Input: part model. Units: mm. Frame: model coordinates. A direction names the side the tool comes from. Give positions to 0.01 mm unless a question says otherwise; leave off trailing zeros. Order: outer loops, then holes, each group sorted by start corner. A loop starts at its lowest first (then second) coordinate and runs counter-clockwise, first axis right, second up. Notation, with made-up numbers: M -10.5,24 L 4.5,24 A31 cw 4.5,60 Z; hole C 60.5,29.5 d2. An arc over 180 degrees is marked long. Use a Markdown table: item, result.
from build123d import *

# Parameters (mm, degrees)
F0_W     = 45
F0_H     = 131
F1_DEPTH = 2
F2_W     = 45
F2_H     = 131
F3_DEPTH = 5
F5_W     = 35
F5_H     = 100
F6_DEPTH = 4
F7_W     = 5
F7_H     = 100
F8_DEPTH = 2
F4_W     = 15
F4_H     = 90
F9_DEPTH = 7.001


with BuildPart() as f1:
    # F0 (on Top) → F1 (new body)
    with BuildSketch(Plane.XY):
        with Locations((22.5, 65.5)):
            Rectangle(F0_W, F0_H)
    extrude(amount=F1_DEPTH)

    # F2 (on face) → F3 (join)
    with BuildSketch(Plane.XY.offset(2)):
        with Locations((22.5, 65.5)):
            Rectangle(F2_W, F2_H)
    extrude(amount=F3_DEPTH)

    # F5 (on face) → F6 (cut)
    with BuildSketch(Plane.XY.offset(7)):
        with Locations((22.5, 71)):
            Rectangle(F5_W, F5_H)
    extrude(amount=-F6_DEPTH, mode=Mode.SUBTRACT)

    # F7 (on face) → F8 (join)
    with BuildSketch(Plane.XY.offset(3)):
        with Locations((22.5, 71)):
            Rectangle(F7_W, F7_H)
    extrude(amount=F8_DEPTH)

    # F4 (on face) → F9 (cut, through all)
    with BuildSketch(Plane.XY.offset(7)):
        with Locations((22.5, 71)):
            Rectangle(F4_W, F4_H)
    extrude(amount=-F9_DEPTH, mode=Mode.SUBTRACT)


solid = f1.part
1) First-contact query: pin 1 Ø12 at (x, y) = (33, 68.5) entering from +Z; pin 2 Ø4 at (x, y) = (23.5, 118) entering from +Z. Flat tips, straight axial feed; report the tip coordinate or a pass-through.
Response values:
| item | result |
|---|---|
| pin 1 | stops at z = 3 |
| pin 2 | stops at z = 5 |
2) Material intervals for line 1 (X direction, y = 118.5, z = 4); line 2 (X direction, y = 102.5, z = 1.75); line 3 (Y direction, x = 22.5, z = 6.5), sorted ascending. Write a range as from..to.
Response values:
| item | result |
|---|---|
| line 1 | x = 0..5, 20..25, 40..45 |
| line 2 | x = 0..15, 30..45 |
| line 3 | y = 0..21, 121..131 |
3) Cut plane A-A on x = 28.5. Return loops of the section in (y, z), and give its area (3 significant figures).
Response values:
| item | result |
|---|---|
| outline | M 0,0 L 26,0 L 26,3 L 21,3 L 21,7 L 0,7 Z; M 116,0 L 131,0 L 131,7 L 121,7 L 121,3 L 116,3 Z |
| area | 247 mm² |
4) Cut plane B-B on y = 93. Return loops of the section in (x, z).
Response values:
| item | result |
|---|---|
| outline | M 0,0 L 15,0 L 15,3 L 5,3 L 5,7 L 0,7 Z; M 30,0 L 45,0 L 45,7 L 40,7 L 40,3 L 30,3 Z |
5) Mould query, pull axis Y, two halves, no side actions, for faces 4 (the face through (22, 0, 3)), 5 (the face through (11, 72, 3)), 6 (the face through (22, 131, 3)). Classes: released by +Y, released by -Y, zero draft, split by the parting line, or undercut.
Response values:
| item | result |
|---|---|
| face 4 | released by -Y |
| face 5 | undercut |
| face 6 | released by +Y |
6) Reachability of faces 1 (the face through (12, 66, 0)), 2 (the face through (22, 116, 2)), 3 (the face through (22.3, 121, 5.5)) from +Z, -Z, +X, -X, +Y, -Y: full face, straight path, thin tool, end or side. Return the list, or none.
Response values:
| item | result |
|---|---|
| face 1 | -Z, +X, -X, +Y, -Y |
| face 2 | +Z, -Z |
| face 3 | +Z |
